Autodesk Inventor part; units mm, degrees
ref_plane "YZ Plane" through (0, 0, 0) normal (1, 0, 0) x (0, 1, 0)
ref_plane "XZ Plane" through (0, 0, 0) normal (0, 1, 0) x (-1, 0, 0)
ref_plane "XY Plane" through (0, 0, 0) normal (0, 0, 1) x (1, 0, 0)
sketch "Sketch1" plane through (0, 0, 0) normal (0, 0, 1) x (1, 0, 0)
  line L0 (-18.875, 7.375) -> (18.875, 7.375)
  line L1 (18.875, 7.375) -> (18.875, -7.375)
  line L2 (18.875, -7.375) -> (-18.875, -7.375)
  line L3 (-18.875, -7.375) -> (-18.875, 7.375)
  line L4 (-18.875, 7.375) -> (18.875, -7.375) construction
  line L5 (18.875, 7.375) -> (-18.875, -7.375) construction
  point P0 (0, 0)
  dimension "d0" = 37.75
  dimension "d1" = 14.75
extrude "Extrusion1" add sketch "Sketch1" along normal blind 3
sketch "Sketch2" plane through (0, 0, 3) normal (0, 0, 1) x (1, 0, 0)
  line L0 (-18.875, -7.375) -> (18.875, -7.375)
  line L1 (18.875, -7.375) -> (18.875, 7.375)
  line L2 (18.875, 7.375) -> (-18.875, 7.375)
  line L3 (-18.875, 7.375) -> (-18.875, -7.375)
  line L4 (-20, 8.5) -> (20, 8.5)
  line L5 (20, 8.5) -> (20, -8.5)
  line L6 (20, -8.5) -> (-20, -8.5)
  line L7 (-20, -8.5) -> (-20, 8.5)
  line L8 (-20, 8.5) -> (20, -8.5) construction
  line L9 (20, 8.5) -> (-20, -8.5) construction
  point P0 (0, 0)
  dimension "d4" = 40
  dimension "d5" = 17
extrude "Extrusion2" add sketch "Sketch2" along normal blind 0.5 contours L3 L2 L1 L0 | L4 L5 L6 L7
sketch "Sketch3" plane through (0, 0, 3.5) normal (0, 0, 1) x (1, 0, 0)
  line L0 (-20, -8.5) -> (20, -8.5)
  line L1 (20, -8.5) -> (20, 8.5)
  line L2 (20, 8.5) -> (-20, 8.5)
  line L3 (-20, 8.5) -> (-20, -8.5)
  line L4 (20, 8.5) -> (-20, 8.5)
  line L5 (-2, 0) -> (2, 0)
  line L6 (2, 0) -> (2, 8.5)
  line L7 (2, 8.5) -> (-2, 8.5)
  line L8 (-2, 8.5) -> (-2, 0)
  line L9 (0, -11.9) -> (0, 11.9)
  line L10 (-28, 0) -> (28, 0)
  point P0 (0, 0)
  dimension "d8" = 4
extrude "Extrusion3" cut sketch "Sketch3" against normal through all contours L9 L2 L6 L5 | L5 L8 L2 L9
fillet "Fillet1" radius 2 2 edges at (-2, 0, 1.75) (2, 0, 1.75)
equation "\"BendRadius\" = Thickness"
equation "\"BendReliefWidth\" = Thickness"
equation "\"BendReliefDepth\" = 0.5 * Thickness"
equation "\"CornerReliefSize\" = 4 * Thickness"
equation "\"MinimumRemnant\" = 2 * Thickness"
equation "\"TransitionRadius\" = BendRadius"
equation "\"JacobiRadiusSize\" = BendRadius"
equation "\"GapSize\" = Thickness"
properties part number "_3DPrint"
Here's how the part is built. I have some questions about the finished solid (model axes, mm). A direction names the side the tool comes from. Coordinates: 2 decimals unless noted, no trailing zeros. Loops run counter-clockwise (first coordinate to the right, second up) from the corner with the lowest first, then second, coordinate; pieces in that order, holes last.
1. Imagine slicing it at D-D, the plane x = -0.5. Please give me the cut outline in (y, z) (3 decimals), and give its area (3 significant figures).
2. For P1, Ø2, axis at x = 7, z = 0.5, coming from the -Y side (3 decimals); P2, Ø1, axis at y = -2.5, z = 0.5, coming from the +X side (3 decimals); P3, Ø0.9, axis at x = 7.5, z = 1, coming from the +Y side (3 decimals), each with a flat end and sliding along its axis, tell me the tip position at first contact or that it passes through.
3. I need wall thicknesses on L1, parallel to X at y = 3, z = 2.1 (3 decimals); L2, parallel to Y at x = 8, z = 1.1 (3 decimals); L3, parallel to X at y = -3.25, z = 1.9 (3 decimals). Which ranges of each line are inside material? Lowest first, please.
4. Imagine slicing it at A-A, the plane x = 10.5. Please give me the cut outline in (y, z) (3 decimals), and give its area (4 significant figures).
5. If we mould it in two halves opening along X, with no side actions, what happens to faces 4 (the flat face through (0, -7.375, 1)), 5 (the cylindrical face through (1.43, 0.6, 1.73)), 6 (the cylindrical face through (-1.4, 0.57, 1.73)), 7 (the flat face through (-18.875, 0, 1))? For each: pulls with the +X half, pulls with the -X half, needs draft (parallel to the pull), parting line crosses it, or undercut.
6. For faces 1 (the flat face through (10, 7.375, 1)), 2 (the flat face through (18.875, 0, 1)), 3 (the flat face through (-2, 5, 2)), which set-ups out of +Z, -Z, +X, -X, +Y, -Y let a thin tool reach every point of the face, with its end or its side?
7. Imagine slicing it at B-B, the plane y = -1. Please give me the cut outline in (x, z) (3 decimals).
Taken from the geometry:
1. outline: (-8.5, 3) - (-7.375, 3) - (-7.375, 0) - (0.063, 0) - (0.063, 3.5) - (-8.5, 3.5) - close
1. area: 26.6 mm2
2. P1: stops at y = -7.375
2. P2: stops at x = 18.875
2. P3: stops at y = 7.375
3. L1: x = -18.875 to -2, 2 to 18.875
3. L2: y = -7.375 to 7.375
3. L3: x = -18.875 to 18.875
4. outline: (-8.5, 3) - (-7.375, 3) - (-7.375, 0) - (7.375, 0) - (7.375, 3) - (8.5, 3) - (8.5, 3.5) - (-8.5, 3.5) - close
4. area: 52.75 mm2
5. face 4: needs draft
5. face 5: undercut
5. face 6: undercut
5. face 7: pulls with the -X half
6. face 1: -Z, +X, -X, +Y
6. face 2: -Z, +X, +Y, -Y
6. face 3: +Z, -Z, +Y
7. outline: (-20, 3) - (-18.875, 3) - (-18.875, 0) - (18.875, 0) - (18.875, 3) - (20, 3) - (20, 3.5) - (-20, 3.5) - close
